Geometry check sheet. Reference: the model listing, model coordinates, mm. Face numbers are marked on the shaded views. Coordinates: 2 decimals unless noted, no trailing zeros. Put each result on its own line as item: value.
from build123d import *

# Parameters (mm, degrees)
SKETCH2_R                                      = 63
BOSS_EXTRUDE1_DEPTH                            = 10
SKETCH4_R                                      = 25
CUT_EXTRUDE1_DEPTH                             = 11
CIRPATTERN1_COUNT                              = 6
CBORE_FOR_M3_SOCKET_HEAD_CAP_SCREW2_AT_2_COUNT = 2
CBORE_FOR_M3_SOCKET_HEAD_CAP_SCREW2_AT_2_PITCH = 12.095599965
CBORE_FOR_M3_SOCKET_HEAD_CAP_SCREW2_AT_3_COUNT = 2
CBORE_FOR_M3_SOCKET_HEAD_CAP_SCREW2_AT_3_PITCH = 23.726372807
CBORE_FOR_M3_SOCKET_HEAD_CAP_SCREW2_AT_4_COUNT = 2
CBORE_FOR_M3_SOCKET_HEAD_CAP_SCREW2_AT_4_PITCH = 34.445354447
CBORE_FOR_M3_SOCKET_HEAD_CAP_SCREW2_AT_5_COUNT = 2
CBORE_FOR_M3_SOCKET_HEAD_CAP_SCREW2_AT_5_PITCH = 43.840620434
CBORE_FOR_M3_SOCKET_HEAD_CAP_SCREW2_AT_6_COUNT = 2
CBORE_FOR_M3_SOCKET_HEAD_CAP_SCREW2_AT_6_PITCH = 51.551115963
CBORE_FOR_M3_SOCKET_HEAD_CAP_SCREW2_AT_7_COUNT = 2
CBORE_FOR_M3_SOCKET_HEAD_CAP_SCREW2_AT_7_PITCH = 57.280531016
CBORE_FOR_M3_SOCKET_HEAD_CAP_SCREW2_AT_8_COUNT = 2
CBORE_FOR_M3_SOCKET_HEAD_CAP_SCREW2_AT_8_PITCH = 60.808687385
CBORE_FOR_M3_SOCKET_HEAD_CAP_SCREW2_AT_9_COUNT = 2
CBORE_FOR_M3_SOCKET_HEAD_CAP_SCREW2_AT_9_PITCH = 62
CBORE_FOR_M3_SOCKET_HEAD_CAP_SCREW2_AT_1_COUNT = 2
CBORE_FOR_M3_SOCKET_HEAD_CAP_SCREW2_AT_1_PITCH = 60.808687385
CBORE_FOR_M3_SOCKET_HEAD_CAP_SCREW2_2_COUNT    = 2
CBORE_FOR_M3_SOCKET_HEAD_CAP_SCREW2_2_PITCH    = 57.280531016
CBORE_FOR_M3_SOCKET_HEAD_CAP_SCREW2_3_COUNT    = 2
CBORE_FOR_M3_SOCKET_HEAD_CAP_SCREW2_3_PITCH    = 51.551115963
CBORE_FOR_M3_SOCKET_HEAD_CAP_SCREW2_4_COUNT    = 2
CBORE_FOR_M3_SOCKET_HEAD_CAP_SCREW2_4_PITCH    = 43.840620434
CBORE_FOR_M3_SOCKET_HEAD_CAP_SCREW2_5_COUNT    = 2
CBORE_FOR_M3_SOCKET_HEAD_CAP_SCREW2_5_PITCH    = 34.445354447
CBORE_FOR_M3_SOCKET_HEAD_CAP_SCREW2_6_COUNT    = 2
CBORE_FOR_M3_SOCKET_HEAD_CAP_SCREW2_6_PITCH    = 23.726372807
CBORE_FOR_M3_SOCKET_HEAD_CAP_SCREW2_7_COUNT    = 2
CBORE_FOR_M3_SOCKET_HEAD_CAP_SCREW2_7_PITCH    = 12.095599965
CHAMFER1_SIZE                                  = 1


with BuildPart() as part:
    # Sketch2 → Boss-Extrude1 (new body)
    with BuildSketch(Plane.XY):
        with Locations((-200, 0)):
            Circle(SKETCH2_R)
    extrude(amount=BOSS_EXTRUDE1_DEPTH)

    # Sketch4 → Cut-Extrude1 (cut, through all)
    with BuildSketch(Plane.XY.offset(10)):
        with Locations((-200, 0)):
            Circle(SKETCH4_R)
    extrude(amount=-CUT_EXTRUDE1_DEPTH, mode=Mode.SUBTRACT)

    # Sketch6 → CBORE for M8 Socket Head Cap Screw1 (revolve, cut)
    with BuildSketch(Plane(origin=(-200, 52.5, 10), x_dir=(0, -1, 0), z_dir=(1, 0, 0))):
        Polygon((0, 0), (0, 19), (3.3, 17.017159957), (3.3, 6), (5.5, 6), (5.5, 0.025), (5.525, 0), align=None)
    cbore_for_m8_socket_head_cap_screw1 = revolve(axis=Axis((-200, 52.5, 16.35), (0, 0, -1)), mode=Mode.SUBTRACT)

    # CirPattern1: CBORE for M8 Socket Head Cap Screw1 ×6 about axis
    cirpattern1_axis = Axis((-200, 0, 0), (0, 0, 1))
    for i in range(1, CIRPATTERN1_COUNT):
        add(cbore_for_m8_socket_head_cap_screw1.rotate(cirpattern1_axis, i * 360 / CIRPATTERN1_COUNT), mode=Mode.SUBTRACT)

    # Sketch11 → CBORE for M3 Socket Head Cap Screw2 (revolve, cut)
    with BuildSketch(Plane(origin=(-200, 31, 0), x_dir=(0, 1, 0), z_dir=(1, 0, 0))):
        Polygon((0, 0), (0, 10), (1.7, 10), (1.7, 3), (3.25, 3), (3.25, 0.025), (3.275, 0), align=None)
    cbore_for_m3_socket_head_cap_screw2 = revolve(axis=Axis((-200, 31, -6.35), (0, 0, 1)), mode=Mode.SUBTRACT)

    # CBORE for M3 Socket Head Cap Screw2 at 2: CBORE for M3 Socket Head Cap Screw2 ×2
    with Locations(*[Vector(0.98078528, -0.195090322, 0) * (i * CBORE_FOR_M3_SOCKET_HEAD_CAP_SCREW2_AT_2_PITCH) for i in range(1, CBORE_FOR_M3_SOCKET_HEAD_CAP_SCREW2_AT_2_COUNT)]):
        add(cbore_for_m3_socket_head_cap_screw2, mode=Mode.SUBTRACT)

    # CBORE for M3 Socket Head Cap Screw2 at 3: CBORE for M3 Socket Head Cap Screw2 ×2
    with Locations(*[Vector(0.923879533, -0.382683432, 0) * (i * CBORE_FOR_M3_SOCKET_HEAD_CAP_SCREW2_AT_3_PITCH) for i in range(1, CBORE_FOR_M3_SOCKET_HEAD_CAP_SCREW2_AT_3_COUNT)]):
        add(cbore_for_m3_socket_head_cap_screw2, mode=Mode.SUBTRACT)

    # CBORE for M3 Socket Head Cap Screw2 at 4: CBORE for M3 Socket Head Cap Screw2 ×2
    with Locations(*[Vector(0.831469612, -0.555570233, 0) * (i * CBORE_FOR_M3_SOCKET_HEAD_CAP_SCREW2_AT_4_PITCH) for i in range(1, CBORE_FOR_M3_SOCKET_HEAD_CAP_SCREW2_AT_4_COUNT)]):
        add(cbore_for_m3_socket_head_cap_screw2, mode=Mode.SUBTRACT)

    # CBORE for M3 Socket Head Cap Screw2 at 5: CBORE for M3 Socket Head Cap Screw2 ×2
    with Locations(*[Vector(0.707106781, -0.707106781, 0) * (i * CBORE_FOR_M3_SOCKET_HEAD_CAP_SCREW2_AT_5_PITCH) for i in range(1, CBORE_FOR_M3_SOCKET_HEAD_CAP_SCREW2_AT_5_COUNT)]):
        add(cbore_for_m3_socket_head_cap_screw2, mode=Mode.SUBTRACT)

    # CBORE for M3 Socket Head Cap Screw2 at 6: CBORE for M3 Socket Head Cap Screw2 ×2
    with Locations(*[Vector(0.555570233, -0.831469612, 0) * (i * CBORE_FOR_M3_SOCKET_HEAD_CAP_SCREW2_AT_6_PITCH) for i in range(1, CBORE_FOR_M3_SOCKET_HEAD_CAP_SCREW2_AT_6_COUNT)]):
        add(cbore_for_m3_socket_head_cap_screw2, mode=Mode.SUBTRACT)

    # CBORE for M3 Socket Head Cap Screw2 at 7: CBORE for M3 Socket Head Cap Screw2 ×2
    with Locations(*[Vector(0.382683432, -0.923879533, 0) * (i * CBORE_FOR_M3_SOCKET_HEAD_CAP_SCREW2_AT_7_PITCH) for i in range(1, CBORE_FOR_M3_SOCKET_HEAD_CAP_SCREW2_AT_7_COUNT)]):
        add(cbore_for_m3_socket_head_cap_screw2, mode=Mode.SUBTRACT)

    # CBORE for M3 Socket Head Cap Screw2 at 8: CBORE for M3 Socket Head Cap Screw2 ×2
    with Locations(*[Vector(0.195090322, -0.98078528, 0) * (i * CBORE_FOR_M3_SOCKET_HEAD_CAP_SCREW2_AT_8_PITCH) for i in range(1, CBORE_FOR_M3_SOCKET_HEAD_CAP_SCREW2_AT_8_COUNT)]):
        add(cbore_for_m3_socket_head_cap_screw2, mode=Mode.SUBTRACT)

    # CBORE for M3 Socket Head Cap Screw2 at 9: CBORE for M3 Socket Head Cap Screw2 ×2
    with Locations(*[(0, -i * CBORE_FOR_M3_SOCKET_HEAD_CAP_SCREW2_AT_9_PITCH, 0) for i in range(1, CBORE_FOR_M3_SOCKET_HEAD_CAP_SCREW2_AT_9_COUNT)]):
        add(cbore_for_m3_socket_head_cap_screw2, mode=Mode.SUBTRACT)

    # CBORE for M3 Socket Head Cap Screw2 at 1: CBORE for M3 Socket Head Cap Screw2 ×2
    with Locations(*[Vector(-0.195090322, -0.98078528, 0) * (i * CBORE_FOR_M3_SOCKET_HEAD_CAP_SCREW2_AT_1_PITCH) for i in range(1, CBORE_FOR_M3_SOCKET_HEAD_CAP_SCREW2_AT_1_COUNT)]):
        add(cbore_for_m3_socket_head_cap_screw2, mode=Mode.SUBTRACT)

    # CBORE for M3 Socket Head Cap Screw2  2: CBORE for M3 Socket Head Cap Screw2 ×2
    with Locations(*[Vector(-0.382683432, -0.923879533, 0) * (i * CBORE_FOR_M3_SOCKET_HEAD_CAP_SCREW2_2_PITCH) for i in range(1, CBORE_FOR_M3_SOCKET_HEAD_CAP_SCREW2_2_COUNT)]):
        add(cbore_for_m3_socket_head_cap_screw2, mode=Mode.SUBTRACT)

    # CBORE for M3 Socket Head Cap Screw2  3: CBORE for M3 Socket Head Cap Screw2 ×2
    with Locations(*[Vector(-0.555570233, -0.831469612, 0) * (i * CBORE_FOR_M3_SOCKET_HEAD_CAP_SCREW2_3_PITCH) for i in range(1, CBORE_FOR_M3_SOCKET_HEAD_CAP_SCREW2_3_COUNT)]):
        add(cbore_for_m3_socket_head_cap_screw2, mode=Mode.SUBTRACT)

    # CBORE for M3 Socket Head Cap Screw2  4: CBORE for M3 Socket Head Cap Screw2 ×2
    with Locations(*[Vector(-0.707106781, -0.707106781, 0) * (i * CBORE_FOR_M3_SOCKET_HEAD_CAP_SCREW2_4_PITCH) for i in range(1, CBORE_FOR_M3_SOCKET_HEAD_CAP_SCREW2_4_COUNT)]):
        add(cbore_for_m3_socket_head_cap_screw2, mode=Mode.SUBTRACT)

    # CBORE for M3 Socket Head Cap Screw2  5: CBORE for M3 Socket Head Cap Screw2 ×2
    with Locations(*[Vector(-0.831469612, -0.555570233, 0) * (i * CBORE_FOR_M3_SOCKET_HEAD_CAP_SCREW2_5_PITCH) for i in range(1, CBORE_FOR_M3_SOCKET_HEAD_CAP_SCREW2_5_COUNT)]):
        add(cbore_for_m3_socket_head_cap_screw2, mode=Mode.SUBTRACT)

    # CBORE for M3 Socket Head Cap Screw2  6: CBORE for M3 Socket Head Cap Screw2 ×2
    with Locations(*[Vector(-0.923879533, -0.382683432, 0) * (i * CBORE_FOR_M3_SOCKET_HEAD_CAP_SCREW2_6_PITCH) for i in range(1, CBORE_FOR_M3_SOCKET_HEAD_CAP_SCREW2_6_COUNT)]):
        add(cbore_for_m3_socket_head_cap_screw2, mode=Mode.SUBTRACT)

    # CBORE for M3 Socket Head Cap Screw2  7: CBORE for M3 Socket Head Cap Screw2 ×2
    with Locations(*[Vector(-0.98078528, -0.195090322, 0) * (i * CBORE_FOR_M3_SOCKET_HEAD_CAP_SCREW2_7_PITCH) for i in range(1, CBORE_FOR_M3_SOCKET_HEAD_CAP_SCREW2_7_COUNT)]):
        add(cbore_for_m3_socket_head_cap_screw2, mode=Mode.SUBTRACT)

    # Chamfer1
    chamfer1_edges = [part.edges().sort_by_distance(p)[0] for p in [
        (-263, 0, 0),
        (-263, 0, 10),
    ]]
    chamfer(chamfer1_edges, length=CHAMFER1_SIZE)


solid = part.part
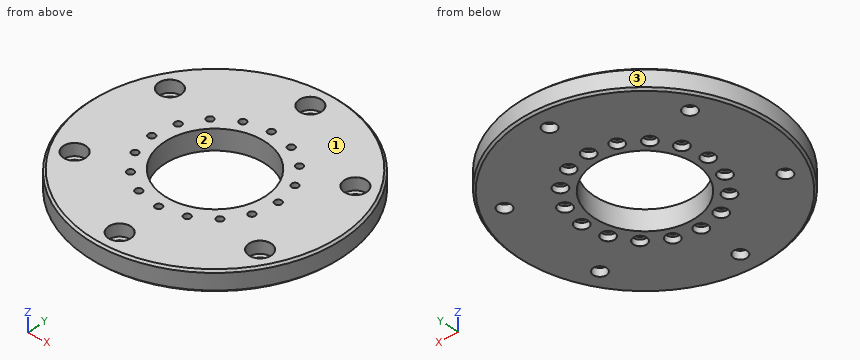
Q1. Draft check along Y on the marked faces 1, 2 and 3. Enter one of: pulls with the +Y half, pulls with the -Y half, needs draft (parallel to the pull), parting line crosses it, or undercut.
Answer block:
face 1: needs draft
face 2: undercut
face 3: parting line crosses it
Q2. Thickness scan on L1, parallel to Y at x = -221, z = 5.5; L2, parallel to X at y = -28.5, z = 9.5; L3, parallel to Y at x = -198, z = 4.5. Record the ranges inside material, lowest first. Write a range as [from, to].
Answer block:
L1: y = [-59.4, -23.35], [-20.49, -13.56], [13.56, 20.49], [23.35, 59.4]
L2: x = [-255.62, -250.49], [-240.45, -213.56], [-210.17, -189.83], [-186.44, -159.55], [-149.51, -144.38]
L3: y = [-62.97, -57.62], [-47.38, -24.92], [24.92, 47.38], [57.62, 62.97]
Q3. Section check A-A on y = 0. State how many separate pieces and enclosed holes the cut face has, then the cut area to 3 significant figures.
Answer block:
separate pieces: 4
enclosed holes: 0
area: 671 mm^2
Q4. Depth check by flat-ended pin: pin 1 Ø4 at (x, y) = (-154.53, -26.25) entering from +Z; pin 2 Ø5.5 at (x, y) = (-231, 0) entering from -Z; pin 3 Ø3 at (y, z) = (-22.5, 4.5) entering from +X; pin 4 Ø6 at (y, z) = (10.5, 1.5) entering from -X. Enter the tip coordinate at first touch or a pass-through.
Answer block:
pin 1: passes through
pin 2: stops at z = 3
pin 3: stops at x = -140.6
pin 4: stops at x = -262.55
